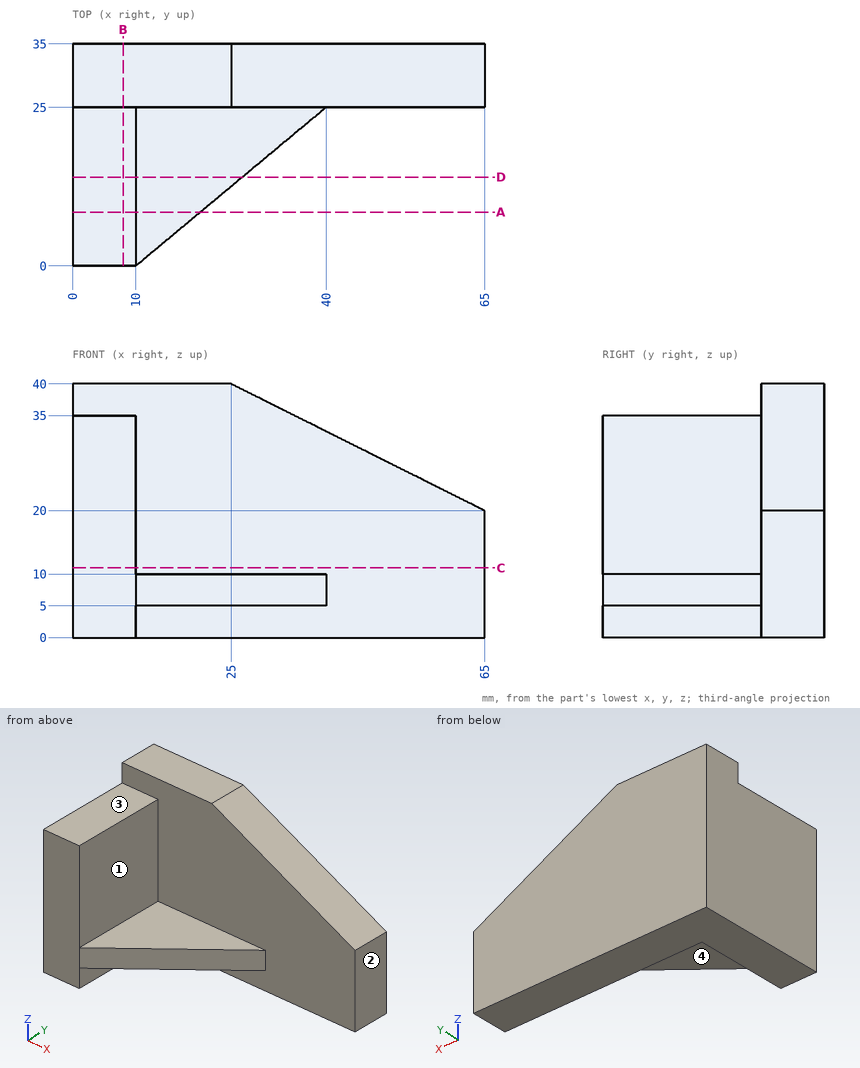
The drawing under review shows one solid part. Ordinate dimensions are in mm from its lowest x, y, z. A direction names the side the tool comes from. Coordinates: 2 decimals unless noted, no trailing zeros. Write each loop counter-clockwise with the first axis right and the second up, starting at its lowest first coordinate (ties: lowest second). Pieces come first, ordered by that corner, then holes. Notation, with made-up numbers: M -35,-8 L -13,-8 A20 cw -13,9 Z; hole C 67,66 d4. An arc over 180 degrees is marked long. Answer as a JSON object with one key per item and string values.
Item 1: Add section D-D, the plane y = 14. Give the boundary of the cut face in (x, z), and give its area (3 significant figures).
Outcome:
{"outline": "M 0,0 L 10,0 L 10,5 L 26.8,5 L 26.8,10 L 10,10 L 10,35 L 0,35 Z", "area": "434 mm²"}
Item 2: Add section C-C, the plane z = 11. Give the boundary of the cut face in (x, y).
Outcome:
{"outline": "M 0,0 L 10,0 L 10,25 L 65,25 L 65,35 L 0,35 Z"}
Item 3: Insertion check: pin 1 Ø20 at (x, z) = (45.5, 23) entering from -Y; pin 2 Ø12 at (x, z) = (23.5, 9.5) entering from -Y; pin 3 Ø7.5 at (x, y) = (32, 13) entering from -Z; pin 4 Ø5 at (x, y) = (4.5, 18.5) entering from +Z. Each pin has a flat end and moves straight along its axis. Give the tip position at first contact, or say it passes through.
Outcome:
{"pin 1": "y = 25", "pin 2": "y = 6.25", "pin 3": "through", "pin 4": "z = 35"}
Item 4: Add section A-A, the plane y = 8.5. Give the boundary of the cut face in (x, z), and give its area (3 significant figures).
Outcome:
{"outline": "M 0,0 L 10,0 L 10,5 L 20.2,5 L 20.2,10 L 10,10 L 10,35 L 0,35 Z", "area": "401 mm²"}
Item 5: Add section B-B, the plane x = 8. Give the boundary of the cut face in (y, z).
Outcome:
{"outline": "M 0,0 L 35,0 L 35,40 L 25,40 L 25,35 L 0,35 Z"}
Item 6: Wall thickness on probe 1 along Y at (x, z) = (46, 25); probe 2 along X at (y, z) = (2, 26); probe 3 along Z at (x, y) = (20, 12): over which ranges is each line inside the solid? List them lowest first.
Outcome:
{"probe 1": "25 to 35", "probe 2": "0 to 10", "probe 3": "5 to 10"}
Item 7: Machinability: for the marked faces 1, 2, 3 and 4, which of the approach directions +Z, -Z, +X, -X, +Y, -Y give a long, thin tool a straight path to every point of the face, cutting with its end or side? Answer none if there is none.
Outcome:
{"face 1": "+Z, +X, -Y", "face 2": "+Z, -Z, +X, +Y, -Y", "face 3": "+Z, +X, -X, -Y", "face 4": "-Z, +X, -Y"}
